```python
from build123d import *

# Parameters (mm, degrees)
SKETCH1_W           = 79
SKETCH1_H           = 51
BOSS_EXTRUDE1_DEPTH = 28.5
SKETCH2_W           = 43.8
SKETCH2_H           = 12.5
BOSS_EXTRUDE2_DEPTH = 15
CUT_EXTRUDE1_DEPTH  = 52
SKETCH4_R           = 1.5
CUT_EXTRUDE2_DEPTH  = 15
SKETCH5_R           = 1.5
CUT_EXTRUDE3_DEPTH  = 15


with BuildPart() as part:
    # Sketch1 → Boss-Extrude1 (new body)
    with BuildSketch(Plane(origin=(0, 0, 0), x_dir=(1, 0, 0), z_dir=(0, 1, 0))):
        Rectangle(SKETCH1_W, SKETCH1_H)
    extrude(amount=BOSS_EXTRUDE1_DEPTH)

    # Sketch2 → Boss-Extrude2 (add)
    with BuildSketch(Plane.ZY.offset(39.5)):
        with Locations((-3.6, 11.25)):
            Rectangle(SKETCH2_W, SKETCH2_H)
    extrude(amount=BOSS_EXTRUDE2_DEPTH)

    # Sketch3 → Cut-Extrude1 (cut, through all)
    with BuildSketch(Plane.XY.offset(25.5)):
        Polygon((-39.5, 28.5), (-39.5, 22.5), (-33.5, 28.5), align=None)
    extrude(amount=-CUT_EXTRUDE1_DEPTH, mode=Mode.SUBTRACT)

    # Sketch4 → Cut-Extrude2 (cut)
    with BuildSketch(Plane.XY.offset(25.5)):
        with Locations((-29.5, 14)):
            Circle(SKETCH4_R)
        with Locations((37, 14)):
            Circle(SKETCH4_R)
    extrude(amount=-CUT_EXTRUDE2_DEPTH, mode=Mode.SUBTRACT)

    # Sketch5 → Cut-Extrude3 (cut)
    with BuildSketch(Plane.XZ):
        with Locations((-26, 0)):
            Circle(SKETCH5_R)
        with Locations((29, 0)):
            Circle(SKETCH5_R)
    extrude(amount=-CUT_EXTRUDE3_DEPTH, mode=Mode.SUBTRACT)


solid = part.part
```
Check sheet for the modelled part. Datum: model origin and axes. Units: mm. A direction names the side the tool comes from. Give positions to 0.01 mm unless a question says otherwise; leave off trailing zeros. Order: outer loops, then holes, each group sorted by start corner. A loop starts at its lowest first (then second) coordinate and runs counter-clockwise, first axis right, second up. Notation, with made-up numbers: M 68.25,67 L 92.25,67 A12 ccw 92.25,83 Z; hole C 20.25,-11 d3. An arc over 180 degrees is marked long. Answer in a Markdown table with one row per item. Add a question column.
Q1. Access from +Z, -Z, +X, -X, +Y, -Y to the whole of each face (thin tool, end or side, straight path). Record for faces 4 (the cylindrical face through (35.8, 13.1, 18.1)), 5 (the flat face through (-47, 5, -4)), 6 (the flat face through (-54.5, 11, -4)), 7 (the flat face through (29, 15, 0)).
Q2. Sectioned sample at A-A, the plane z = 20.5. Record the boundary of the cut face in (x, y).
Q3. Sectioned sample at B-B, the plane y = 7.25. Record the boundary of the cut face in (x, z), and give its area (3 significant figures).
Q4. Thickness scan on L1, parallel to Y at x = 37, z = 21; L2, parallel to Z at x = 29, y = 5; L3, parallel to Y at x = -29, z = 22. Record the ranges inside material, lowest first.
Q5. Sectioned sample at D-D, the plane z = 0. Record the boundary of the cut face in (x, y), and give its area (3 significant figures).
Q6. Gauge pin test, flat ends, axial feed: pin 1 Ø2.5 at (x, z) = (-26, 0) entering from -Y; pin 2 Ø3.5 at (x, y) = (-30, 14) entering from +Z; pin 3 Ø7.5 at (x, z) = (-48.5, -14.5) entering from +Y; pin 4 Ø0.9 at (x, y) = (36.5, 13.5) entering from +Z. Record the tip position at first contact, or that the pin passes through.
Q7. Release check for a two-part mould opening along X. For faces 1 (the flat face through (-47, 11, 18.3)), 2 (the cylindrical face through (-27.5, 7.4, 0.07)), 3 (the flat face through (39.5, 14, 0)) record: released by +X, released by -X, zero draft, split by the parting line, or undercut.
Q8. Sectioned sample at C-C, the plane x = 37. Record the boundary of the cut face in (y, z).
Verdict:
| question | item | result |
|---|---|---|
| 1 | face 4 | +Z |
| 1 | face 5 | +Z, -Z, -X, -Y |
| 1 | face 6 | +Z, -Z, -X, +Y, -Y |
| 1 | face 7 | -Y |
| 2 | outline | M -39.5,0 L 39.5,0 L 39.5,28.5 L -33.5,28.5 L -39.5,22.5 Z; hole C -29.5,14 d3; hole C 37,14 d3 |
| 3 | outline | M -54.5,-25.5 L 39.5,-25.5 L 39.5,25.5 L -39.5,25.5 L -39.5,18.3 L -54.5,18.3 Z; hole C -26,0 d3; hole C 29,0 d3 |
| 3 | area | 4,670 mm² |
| 4 | L1 | 0 to 12.5, 15.5 to 28.5 |
| 4 | L2 | -25.5 to -1.5, 1.5 to 25.5 |
| 4 | L3 | 0 to 12.59, 15.41 to 28.5 |
| 5 | outline | M -54.5,5 L -39.5,5 L -39.5,0 L -27.5,0 L -27.5,15 L -24.5,15 L -24.5,0 L 27.5,0 L 27.5,15 L 30.5,15 L 30.5,0 L 39.5,0 L 39.5,28.5 L -33.5,28.5 L -39.5,22.5 L -39.5,17.5 L -54.5,17.5 Z |
| 5 | area | 2,330 mm² |
| 6 | pin 1 | y = 15 |
| 6 | pin 2 | z = 25.5 |
| 6 | pin 3 | y = 17.5 |
| 6 | pin 4 | z = 10.5 |
| 7 | face 1 | zero draft |
| 7 | face 2 | undercut |
| 7 | face 3 | released by +X |
| 8 | outline | M 0,-25.5 L 28.5,-25.5 L 28.5,25.5 L 15.5,25.5 L 15.5,10.5 L 12.5,10.5 L 12.5,25.5 L 0,25.5 Z |
